Can you work these out from the model? Positions are in its coordinate system, mm. A direction names the side the tool comes from. Give positions to 0.01 mm unless a question says otherwise; leave off trailing zeros. Loops run counter-clockwise (first coordinate to the right, second up) from the corner with the lowest first, then second, coordinate; pieces in that order, holes last. Notation, with made-up numbers: (4.25, -26) - (18.25, -26) arc R17 ccw to (18.25, 2) - close; hole circle Ø8 at (-4, -14). An arc over 180 degrees is marked (long way). Use a Markdown table: item, result. Add a question column.
```python
from build123d import *

# Parameters (mm, degrees)
ESQUISSE3_R                  = 72
BOSS_EXTRU_1_DEPTH           = 40
BOSS_EXTRU_1_TAPER           = 7
CONG_2_R                     = 2
ESQUISSE26_R                 = 7.5
ENL_V_MAT_EXTRU_1_DEPTH      = 4
ESQUISSE39_W                 = 10
ESQUISSE39_H                 = 10
ENL_V_MAT_EXTRU_4_DEPTH      = 20
D_GAGEMENT_M2_51_AT_2_COUNT  = 2
D_GAGEMENT_M2_51_AT_2_PITCH  = 10
R_P_TITION_CIRCULAIRE5_COUNT = 4
D_GAGEMENT_M21_D             = 2.2
D_GAGEMENT_M21_DEPTH         = 7
D_GAGEMENT_M21_TIP           = 0.660946681
ENL_V_MAT_EXTRU_2_DEPTH      = 15
ESQUISSE33_R                 = 2
ENL_V_MAT_EXTRU_3_DEPTH      = 105.608795203
ESQUISSE36_W                 = 10
ESQUISSE36_H                 = 12
PASSAGE_DE_CABLE_DEPTH       = 132.153294527
ETOILE_DEPTH                 = 4


with BuildPart() as part:
    # Esquisse3 → Boss.-Extru.1 (new body)
    with BuildSketch(Plane(origin=(0, 0, 0), x_dir=(1, 0, 0), z_dir=(0, 1, 0))):
        Circle(ESQUISSE3_R)
    extrude(amount=BOSS_EXTRU_1_DEPTH, taper=BOSS_EXTRU_1_TAPER)

    # Congé2
    cong_2_edges = [part.edges().sort_by_distance(p)[0] for p in [
        (-67.088617564, 40, 0),
    ]]
    fillet(cong_2_edges, radius=CONG_2_R)

    # Esquisse26 → Enlèv. mat.-Extru.1 (cut)
    with BuildSketch(Plane(origin=(0, 0, 0), x_dir=(-1, 0, 0), z_dir=(0, -1, 0))):
        with Locations(Location((0, 0, 0), (0, 0, 90))):
            Circle(ESQUISSE26_R)
    extrude(amount=-ENL_V_MAT_EXTRU_1_DEPTH, mode=Mode.SUBTRACT)

    # Esquisse39 → Enlèv. mat.-Extru.4 (cut)
    with BuildSketch(Plane.XZ):
        with Locations((67, 0)):
            Rectangle(ESQUISSE39_W, ESQUISSE39_H)
    enl_v_mat_extru_4 = extrude(amount=-ENL_V_MAT_EXTRU_4_DEPTH, mode=Mode.SUBTRACT)

    # Esquisse42 → Dégagement M2.51 (revolve, cut)
    with BuildSketch(Plane(origin=(62, 15, 0), x_dir=(0, 0, -1), z_dir=(0, 1, 0))):
        Polygon((0, 0), (0, 4.811161836), (1.35, 4), (1.35, 0), align=None)
    d_gagement_m2_51 = revolve(axis=Axis((68.35, 15, 0), (-1, 0, 0)), mode=Mode.SUBTRACT)

    # Dégagement M2.51 at 2: Dégagement M2.51 ×2
    with Locations(*[(0, -i * D_GAGEMENT_M2_51_AT_2_PITCH, 0) for i in range(1, D_GAGEMENT_M2_51_AT_2_COUNT)]):
        add(d_gagement_m2_51, mode=Mode.SUBTRACT)

    # Répétition circulaire5: Enlèv. mat.-Extru.4, Dégagement M2.51 ×4 about axis
    r_p_tition_circulaire5_axis = Axis((0, 0, 0), (0, 1, 0))
    add([enl_v_mat_extru_4.rotate(r_p_tition_circulaire5_axis, i * 360 / R_P_TITION_CIRCULAIRE5_COUNT) for i in range(1, R_P_TITION_CIRCULAIRE5_COUNT)], mode=Mode.SUBTRACT)
    add([d_gagement_m2_51.rotate(r_p_tition_circulaire5_axis, i * 360 / R_P_TITION_CIRCULAIRE5_COUNT) for i in range(1, R_P_TITION_CIRCULAIRE5_COUNT)], mode=Mode.SUBTRACT)

    # Répétition circulaire5 copy 1 sketch → Répétition circulaire5 copy 1 (revolve, cut)
    with BuildSketch(Plane(origin=(0, 5, -62), x_dir=(-1, 0, 0), z_dir=(0, 1, 0))):
        Polygon((0, 0), (0, 4.811161836), (1.35, 4), (1.35, 0), align=None)
    revolve(axis=Axis((0, 5, -68.35), (0, 0, 1)), mode=Mode.SUBTRACT)

    # Répétition circulaire5 copy 2 sketch → Répétition circulaire5 copy 2 (revolve, cut)
    with BuildSketch(Plane(origin=(-62, 5, 0), x_dir=(0, 0, 1), z_dir=(0, 1, 0))):
        Polygon((0, 0), (0, 4.811161836), (1.35, 4), (1.35, 0), align=None)
    revolve(axis=Axis((-68.35, 5, 0), (1, 0, 0)), mode=Mode.SUBTRACT)

    # Répétition circulaire5 copy 3 sketch → Répétition circulaire5 copy 3 (revolve, cut)
    with BuildSketch(Plane(origin=(0, 5, 62), x_dir=(1, 0, 0), z_dir=(0, 1, 0))):
        Polygon((0, 0), (0, 4.811161836), (1.35, 4), (1.35, 0), align=None)
    revolve(axis=Axis((0, 5, 68.35), (0, 0, -1)), mode=Mode.SUBTRACT)

    # Dégagement M21
    with Locations(Plane(origin=(0, 40, 0), x_dir=(1, 0, 0), z_dir=(0, 1, 0))):
        with Locations((7.5, 0), (-7.5, 0)):
            Hole(D_GAGEMENT_M21_D / 2, depth=D_GAGEMENT_M21_DEPTH)
            with Locations((0, 0, -(D_GAGEMENT_M21_DEPTH + D_GAGEMENT_M21_TIP / 2))):  # 118° drill point
                Cone(0, D_GAGEMENT_M21_D / 2, D_GAGEMENT_M21_TIP, mode=Mode.SUBTRACT)

    # Esquisse30 → Enlèv. mat.-Extru.2 (cut)
    with BuildSketch(Plane(origin=(0, 40, 0), x_dir=(1, 0, 0), z_dir=(0, 1, 0))):
        with BuildLine():
            ThreePointArc((-3, 0), (0, -3), (3, 0))
            Line((3, 0), (-3, 0))
        make_face()
        with BuildLine():
            Line((-3, 0), (3, 0))
            ThreePointArc((3, 0), (0, 3), (-3, 0))
        make_face()
    extrude(amount=-ENL_V_MAT_EXTRU_2_DEPTH, mode=Mode.SUBTRACT)

    # Esquisse33 → Enlèv. mat.-Extru.3 (cut, through all)
    with BuildSketch(Plane(origin=(0, 25, 0), x_dir=(1, 0, 0), z_dir=(0, 1, 0))):
        with Locations(Location((0, 0, 0), (0, 0, 270))):
            Circle(ESQUISSE33_R)
    extrude(amount=-ENL_V_MAT_EXTRU_3_DEPTH, mode=Mode.SUBTRACT)

    # Esquisse36 → Passage de cable (cut, through all, along a direction that is not the sketch's normal)
    with BuildSketch(Plane.XZ):
        with Locations((45, 0)):
            Rectangle(ESQUISSE36_W, ESQUISSE36_H)
    extrude(amount=-PASSAGE_DE_CABLE_DEPTH, dir=(0.5522931199127548, -0.8336499923211392, 0), mode=Mode.SUBTRACT)

    # Esquisse38 → Etoile (cut)
    with BuildSketch(Plane(origin=(0, 0, 0), x_dir=(-1, 0, 0), z_dir=(0, -1, 0))):
        with BuildLine():
            Line((17.829336699, 2.851269982), (6.749815306, 4.908311464))
            ThreePointArc((6.749815306, 4.908311464), (5.543319697, 5.543319697), (4.908311464, 6.749815306))
            Line((4.908311464, 6.749815306), (2.851269982, 17.829336699))
            ThreePointArc((2.851269982, 17.829336699), (0, 20.199961), (-2.851269982, 17.829336699))
            Line((-2.851269982, 17.829336699), (-4.908311464, 6.749815306))
            ThreePointArc((-4.908311464, 6.749815306), (-5.543319697, 5.543319697), (-6.749815306, 4.908311464))
            Line((-6.749815306, 4.908311464), (-17.829336699, 2.851269982))
            ThreePointArc((-17.829336699, 2.851269982), (-20.199961, 0), (-17.829336699, -2.851269982))
            Line((-17.829336699, -2.851269982), (-6.749815306, -4.908311464))
            ThreePointArc((-6.749815306, -4.908311464), (-5.543319697, -5.543319697), (-4.908311464, -6.749815306))
            Line((-4.908311464, -6.749815306), (-2.851269982, -17.829336699))
            ThreePointArc((-2.851269982, -17.829336699), (0, -20.199961), (2.851269982, -17.829336699))
            Line((2.851269982, -17.829336699), (4.908311464, -6.749815306))
            ThreePointArc((4.908311464, -6.749815306), (5.543319697, -5.543319697), (6.749815306, -4.908311464))
            Line((6.749815306, -4.908311464), (17.829336699, -2.851269982))
            ThreePointArc((17.829336699, -2.851269982), (20.199961, 0), (17.829336699, 2.851269982))
        make_face()
    extrude(amount=-ETOILE_DEPTH, mode=Mode.SUBTRACT)


solid = part.part
```
1. If we mould it in two halves opening along X, with no side actions, what happens to faces 1 (the face through (66, 10, -5)), 2 (the face through (3.894, 1.972, 12.212)), 3 (the face through (62, 10, 0))? For each: released by +X, released by -X, zero draft, split by the parting line, or undercut.
2. Will these pins go through, and if not, where does the flat tip stop? P1, Ø12, axis at y = 6.5, z = -51.5, coming from the +X side; P2, Ø1.6, axis at x = 0, y = 15, coming from the +Z side; P3, Ø4, axis at x = -50.5, y = 33.5, coming from the +Z side; P4, Ø8.5, axis at x = 65, z = 2.5, coming from the -Y side.
3. Suppose I cut it at A-A (y = 22). List the corners of the cut face in (x, z) for me (3 decimals), and give its area (3 significant figures).
4. Suppose I cut it at B-B (y = 36.5). List the corners of the cut face in (x, z) for me, and give its area (3 significant figures).
5. Please list where these lines run through material, in increasing order: line 1 along Y through (x, z) = (0, -60.9); line 2 along Z through (x, y) = (22, 9.5); line 3 along Z through (x, y) = (60, 5). Write a range as [from, to].
6. On a 3-axis mill with a long thin cutter (end or side, diameter ignored), from which of +Z, -Z, +X, -X, +Y, -Y can I reach the whole of each face in a straight line? I mean faces 4 (the face through (-12.212, 1.972, 3.894)), 5 (the face through (5, 10, -66)), 6 (the face through (26.935, 19.72, -0.084)). Say none if no direction works.
Results below:
| question | item | result |
|---|---|---|
| 1 | face 1 | zero draft |
| 1 | face 2 | undercut |
| 1 | face 3 | released by +X |
| 2 | P1 | x = 54.86 |
| 2 | P2 | z = 57.67 |
| 2 | P3 | z = 47.53 |
| 2 | P4 | y = 0 |
| 3 | outline | circle Ø138.597 at (0, 0); hole circle Ø4 at (0, 0); hole (25.425, -6) - (35.425, -6) - (35.425, 6) - (25.425, 6) - close |
| 3 | area | 15,000 mm² |
| 4 | outline | circle Ø135.04 at (0, 0); hole circle Ø2.2 at (-7.5, 0); hole circle Ø6 at (0, 0); hole circle Ø2.2 at (7.5, 0); hole (15.82, -6) - (25.82, -6) - (25.82, 6) - (15.82, 6) - close |
| 4 | area | 14,200 mm² |
| 5 | line 1 | [0, 3.65], [6.35, 13.65], [16.35, 40] |
| 5 | line 2 | [-67.33, 67.33] |
| 5 | line 3 | [-38.68, -1.35], [1.35, 38.68] |
| 6 | face 4 | -Y |
| 6 | face 5 | -Z, -Y |
| 6 | face 6 | none |
